```python
from build123d import *

# Parameters (mm, degrees)
F1_DEPTH = 10
F3_D     = 6
F5_R     = 4
F6_DEPTH = 30
F7_SIZE  = 6


with BuildPart() as f1:
    # F0 (on Front) → F1 (new body, symmetric)
    with BuildSketch(Plane.XZ):
        with BuildLine():
            ThreePointArc((-3.4641016151, 2), (0, 4), (3.4641016151, 2))
            Line((3.4641016151, 2), (20, 2))
            Line((20, 2), (20, 7))
            Line((20, 7), (-20, 7))
            Line((-20, 7), (-20, 2))
            Line((-20, 2), (-3.4641016151, 2))
        make_face()
        with BuildLine():
            Line((-3.4641016151, 2), (3.4641016151, 2))
            ThreePointArc((3.4641016151, 2), (0, 4), (-3.4641016151, 2))
        make_face()
    extrude(amount=F1_DEPTH, both=True)

    # F3 (through all)
    with Locations(Plane.XY.offset(7)):
        with Locations((15, 0), (-15, 0)):
            Hole(F3_D / 2)

    # F5 (on face) → F6 (cut, symmetric)
    with BuildSketch(Plane(origin=(0, 0, 0), x_dir=(-0.7071067812, 0.7071067812, 0), z_dir=(0.7071067812, 0.7071067812, 0))):
        Circle(F5_R)
    extrude(amount=F6_DEPTH, both=True, mode=Mode.SUBTRACT)

    # F7
    f7_edges = [f1.edges().sort_by_distance(p)[0] for p in [
        (-20, -10, 4.5),
        (20, 10, 4.5),
        (20, -10, 4.5),
        (-20, 10, 4.5),
    ]]
    chamfer(f7_edges, length=F7_SIZE)


solid = f1.part
```
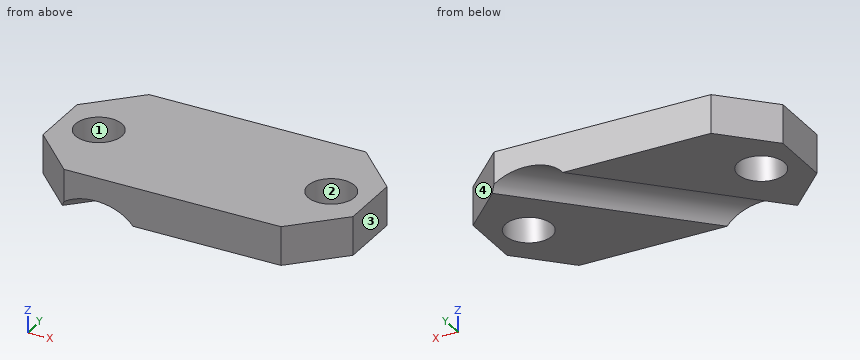
Input: part model. Units: mm. Frame: model coordinates. Face numbers are marked on the shaded views. Round coordinates to 2 decimals unless told otherwise and drop trailing zeros. Order: outer loops, then holes, each group sorted by start corner. A loop starts at its lowest first (then second) coordinate and runs counter-clockwise, first axis right, second up. Notation, with made-up numbers: (40.5, 19) - (48.5, 19) arc R18 cw to (48.5, 53) - close; hole circle Ø7 at (82.5, 57). An arc over 180 degrees is marked (long way). One line per question, with ' | ' between items. Start each with the question number.
1) Ray query, probe 1 along X at (y, z) = (-1.25, 6.35); probe 2 along Y at (x, z) = (-16, 4.7); probe 3 along Z at (x, y) = (-7.5, -7.5). Return the intervals inside material, ascending.
2) Cut plane A-A, the plane x = -15. Return the cut outline in (y, z), then the cut area to 3 significant figures.
3) Cut plane B-B, the plane z = 4.75. Return the cut outline in (x, y).
4) Contact query for flat-ended pins moving along their axis: P1, Ø2, axis at x = 7, y = 4, coming from the -Z side; P2, Ø2, axis at x = 3, y = 3.5, coming from the -Z side; P3, Ø2, axis at x = 5.5, y = 4, coming from the -Z side. Output: stop coordinate, or through.
5) Pull-direction query (Y, two-part tool) for the marked faces 1, 2, 3 and 4; classes: +Y half, -Y half, draft (parallel to the pull), parting line (faces both ways), or undercut.
6) Cut plane C-C, the plane y = 1.25. Give the number of separate pieces and of enclosed holes in the cut face, then the cut area to 3 significant figures.
Worked out:
1) probe 1: x = -20 to -17.73, -12.27 to 12.27, 17.73 to 20 | probe 2: y = -8 to -2.83, 2.83 to 8 | probe 3: z = 4 to 7
2) outline: (-9, 2) - (-3, 2) - (-3, 7) - (-9, 7) - close; (3, 2) - (9, 2) - (9, 7) - (3, 7) - close | area: 60.0 mm^2
3) outline: (-20, -4) - (-14, -10) - (14, -10) - (20, -4) - (20, 4) - (14, 10) - (-14, 10) - (-20, 4) - close; hole circle Ø6 at (-15, 0); hole circle Ø6 at (15, 0)
4) P1: stops at z = 2.5 | P2: stops at z = 3.76 | P3: stops at z = 3.43
5) face 1: undercut | face 2: undercut | face 3: draft | face 4: +Y half
6) separate pieces: 3 | enclosed holes: 0 | area: 132 mm^2
